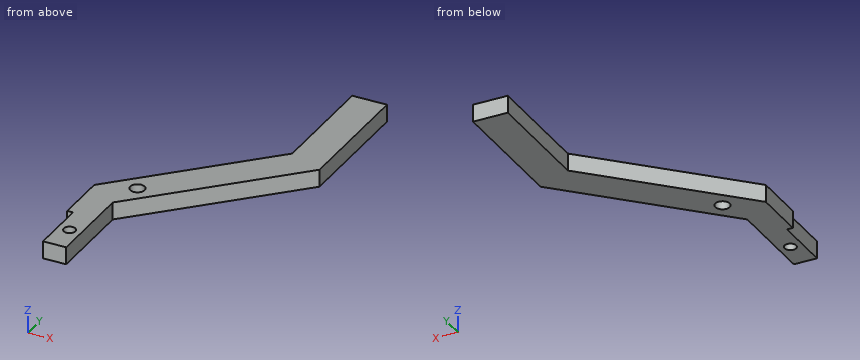
```python
from build123d import *

# Parameters (mm, degrees)
BOSS_EXTRUDE1_DEPTH = 3
SKETCH3_W           = 2
SKETCH3_H           = 10
CUT_EXTRUDE2_DEPTH  = 3
SKETCH5_W           = 1
SKETCH5_H           = 12.104258702
CUT_EXTRUDE4_DEPTH  = 10
SKETCH6_R           = 1.25
CUT_EXTRUDE5_DEPTH  = 3
SKETCH7_R           = 1
CUT_EXTRUDE6_DEPTH  = 10


with BuildPart() as part:
    # Sketch1 → Boss-Extrude1 (new body)
    with BuildSketch(Plane.XY):
        Polygon((-29.183975781, -29.96919486), (-29.183975781, -14.46919486), (-5.683975781, 9.03080514), (-5.683975781, 31.516086514), (-11.683975781, 31.516086514), (-11.683975781, 11.516086514), (-35.183975781, -11.983913486), (-35.183975781, -29.96919486), align=None)
    extrude(amount=BOSS_EXTRUDE1_DEPTH)

    # Sketch3 → Cut-Extrude2 (cut)
    with BuildSketch(Plane.XY.offset(3)):
        with Locations((-34.183975781, -24.96919486)):
            Rectangle(SKETCH3_W, SKETCH3_H)
    extrude(amount=-CUT_EXTRUDE2_DEPTH, mode=Mode.SUBTRACT)

    # Sketch5 → Cut-Extrude4 (cut)
    with BuildSketch(Plane.XY.offset(3)):
        with Locations((-34.683975781, -13.917065509)):
            Rectangle(SKETCH5_W, SKETCH5_H)
    extrude(amount=-CUT_EXTRUDE4_DEPTH, mode=Mode.SUBTRACT)

    # Sketch6 → Cut-Extrude5 (cut)
    with BuildSketch(Plane.XY.offset(3)):
        with Locations((-27.823975781, -8.866554173)):
            Circle(SKETCH6_R)
    extrude(amount=-CUT_EXTRUDE5_DEPTH, mode=Mode.SUBTRACT)

    # Sketch7 → Cut-Extrude6 (cut)
    with BuildSketch(Plane.XY.offset(3)):
        with Locations((-31.183975781, -24.96919486)):
            Circle(SKETCH7_R)
    extrude(amount=-CUT_EXTRUDE6_DEPTH, mode=Mode.SUBTRACT)


solid = part.part
```
Can you work these out from the model? Positions are in its coordinate system, mm. Coordinates: 2 decimals unless noted, no trailing zeros. Order: outer loops, then holes, each group sorted by start corner. A loop starts at its lowest first (then second) coordinate and runs counter-clockwise, first axis right, second up.
1. If we section it at B-B (y = 19.5): Please give me the cut outline in (x, z).
2. If we section it at A-A (z = 0.9): Please give me the cut outline in (x, y), then the cut area to 3 significant figures.
3. I'm going to push flat-ended pins straight in: pin 1 (1 mm diameter, centred on y = -4, z = 0.5, fed in from +X); pin 2 (0.8 mm diameter, centred on x = -34, z = 1, fed in from -Y); pin 3 (0.9 mm diameter, centred on y = -22, z = 2, fed in from +X). Where does each tip first touch, or does it pass through?
4. If we section it at C-C (x = -19.5): Please give me the cut outline in (y, z).
5. I need wall thicknesses on line 1 (X direction, y = 16.5, z = 2.75); line 2 (X direction, y = -16.5, z = 0.6); line 3 (Y direction, x = -18.25, z = 1.8). Which ranges of each line are inside material? Lowest first, please.
Entries:
1. outline: (-11.68, 0) - (-5.68, 0) - (-5.68, 3) - (-11.68, 3) - close
2. outline: (-34.18, -19.97) - (-33.18, -19.97) - (-33.18, -29.97) - (-29.18, -29.97) - (-29.18, -14.47) - (-5.68, 9.03) - (-5.68, 31.52) - (-11.68, 31.52) - (-11.68, 11.52) - (-34.18, -10.98) - close; hole circle Ø2 at (-31.18, -24.97); hole circle Ø2.5 at (-27.82, -8.87)
2. area: 391 mm2
3. pin 1: stops at x = -18.21
3. pin 2: stops at y = -19.97
3. pin 3: stops at x = -29.18
4. outline: (-4.79, 0) - (3.7, 0) - (3.7, 3) - (-4.79, 3) - close
5. line 1: x = -11.68 to -5.68
5. line 2: x = -34.18 to -29.18
5. line 3: y = -3.54 to 4.95
